Autodesk Inventor part; units mm, degrees
ref_plane "YZ Plane" through (0, 0, 0) normal (1, 0, 0) x (0, 1, 0)
ref_plane "XZ Plane" through (0, 0, 0) normal (0, 1, 0) x (-1, 0, 0)
ref_plane "XY Plane" through (0, 0, 0) normal (0, 0, 1) x (1, 0, 0)
sketch "Sketch1" plane through (0, 0, 0) normal (0, 0, 1) x (1, 0, 0)
  line L0 (-7.2739, -1.4271) -> (7.2739, -1.4271)
  line L1 (7.2739, -1.4271) -> (7.2739, 1.4271)
  line L2 (7.2739, 1.4271) -> (-7.2739, 1.4271)
  line L3 (-7.2739, 1.4271) -> (-7.2739, -1.4271)
  line L4 (-7.2739, -1.4271) -> (7.2739, 1.4271) construction
  line L5 (7.2739, -1.4271) -> (-7.2739, 1.4271) construction
  line L6 (9.525, 3.6783) -> (-9.525, 3.6783)
  line L7 (-9.525, 3.6783) -> (-9.525, 6.4723)
  line L8 (-9.525, 6.4723) -> (9.525, 6.4723)
  line L9 (9.525, 6.4723) -> (9.525, 3.6783)
  line L10 (9.525, 3.6783) -> (-9.525, 6.4723) construction
  line L11 (-9.525, 3.6783) -> (9.525, 6.4723) construction
  line L12 (-7.2739, 1.4271) -> (-9.525, 3.6783)
  line L13 (7.2739, 1.4271) -> (9.525, 3.6783)
  line L14 (-10.922, 5.0753) -> (-8.1026, 7.8947)
  line L15 (-10.922, 5.0753) -> (-6.9348, 5.0753) construction
  line L16 (-10.922, 5.0753) -> (-9.525, 3.6783)
  line L17 (10.922, 5.0753) -> (8.1026, 7.8947)
  line L18 (9.525, 3.6783) -> (10.922, 5.0753)
  line L19 (-8.1026, 7.8947) -> (8.1026, 7.8947)
  line L20 (-19.05, -1.4271) -> (19.05, -1.4271)
  line L21 (19.05, -1.4271) -> (19.05, 15.8839)
  line L22 (19.05, 15.8839) -> (-19.05, 15.8839)
  line L23 (-19.05, 15.8839) -> (-19.05, -1.4271)
  point P0 (0, 0)
  point P1 (0, 5.0753)
  point P2 (0, -1.4271)
  dimension "d0" = 135
  dimension "d1" = 135
  dimension "d2" = 19.05
  dimension "d3" = 2.794
  dimension "d4" = 45
  dimension "d5" = 4.2164
  dimension "d6" = 90
  dimension "d7" = 90
  dimension "d8" = 9.3218
  dimension "d9" = 38.1
extrude "Extrusion1" add sketch "Sketch1" against normal blind 177.8 contours L20 L23 L22 L21 L1 L13 L18 L17 L19 L14 L16 L12 L3
sketch "Sketch2" plane through (0, 0, -177.8) normal (0, 0, -1) x (-1, 0, 0)
  arc A0 (19.05, 29.7163) -> (-19.05, 29.7163) centre (0, 29.7163) ccw
  line L0 (19.05, -1.4271) -> (19.05, 15.8839)
  line L1 (19.05, 15.8839) -> (19.05, -1.4271)
  line L2 (19.05, 15.8839) -> (19.05, 29.7163)
  line L3 (-19.05, -1.4271) -> (-19.05, 15.8839)
  line L4 (-19.05, 15.8839) -> (-19.05, 29.7163)
  line L5 (19.05, 15.8839) -> (-19.05, 15.8839)
  point P0 (0, 0)
extrude "Extrusion2" add sketch "Sketch2" against normal blind 50.8
sketch "Sketch3" plane through (0, 0, -177.8) normal (0, 0, -1) x (-1, 0, 0)
  arc A0 (19.05, 29.7163) -> (-19.05, 29.7163) centre (0, 29.7163) ccw
  point P0 (0, 0)
hole "Hole1" at (0, 29.7163, -177.8) direction (0, 0, 1) diameter 21.6 end through all
fillet "Fillet1" radius 3.175 2 edges at (-19.05, 15.8839, -63.5) (19.05, 15.8839, -63.5)
properties part number "Laser mount 7 inches"
Design review of the part built by this model. Coordinates are the model's own, in mm. A direction names the side the tool comes from. Round coordinates to 2 decimals unless told otherwise and drop trailing zeros. Write each loop counter-clockwise with the first axis right and the second up, starting at its lowest first coordinate (ties: lowest second). Pieces come first, ordered by that corner, then holes.
Item 1: For faces 1 (the flat face through (0, 15.884, -63)), 2 (the cylindrical face through (-0.475, 18.927, -152.044)), 3 (the cylindrical face through (18.095, 14.979, -64.389)), 4 (the flat face through (-7.274, 0, -88)), 5 (the cylindrical face through (-18.145, 14.929, -64.389)), list the 3-axis set-ups (+Z, -Z, +X, -X, +Y, -Y) from which the entire face can be reached by the end or side of a thin tool; tool diameter is ignored.
Item 2: Wall thickness on L1, parallel to Y at x = 0, z = -153; L2, parallel to Y at x = 11, z = -78; L3, parallel to Y at x = -5, z = -113: over which ranges is each line inside the solid? List them lowest first.
Item 3: Consider section A-A on x = 0. Give the boundary of the cut face in (y, z).
Item 4: Consider section C-C on y = 36.5. Give the boundary of the cut face in (x, z).
Item 5: Consider section B-B on z = -61.5. Give the boundary of the cut face in (x, y) (3 decimals).
Item 6: For pin 1 Ø9.5 at (x, z) = (-4, -52) entering from +Y; pin 2 Ø11 at (x, y) = (9, 36.5) entering from +Z, all flat-tipped, find the tip position at first contact; note any pin that passes through.
Item 7: Draft analysis for pull direction X (two halves, no side actions). For faces 6 (the flat face through (9, 39, -127)), 7 (the cylindrical face through (-0.42, 48.76, -152.76)), 8 (the flat face through (7.274, 0, -88)), state which applies: released by +X, released by -X, zero draft, split by the parting line, or undercut.
Check values:
1. face 1: +Z, +X, -X, +Y
1. face 2: +Z, -Z
1. face 3: +Z, +X, +Y
1. face 4: +Z, -Z, -Y
1. face 5: +Z, -X, +Y
2. L1: y = 7.89 to 18.92, 40.52 to 48.77
2. L2: y = -1.43 to 15.88
2. L3: y = 7.89 to 15.88
3. outline: (7.89, -177.8) - (18.92, -177.8) - (18.92, -127) - (15.88, -127) - (15.88, 0) - (7.89, 0) - close; (40.52, -177.8) - (48.77, -177.8) - (48.77, -127) - (40.52, -127) - close
4. outline: (-17.8, -177.8) - (-8.4, -177.8) - (-8.4, -127) - (-17.8, -127) - close; (8.4, -177.8) - (17.8, -177.8) - (17.8, -127) - (8.4, -127) - close
5. outline: (-19.05, -1.427) - (-7.274, -1.427) - (-7.274, 1.427) - (-9.525, 3.678) - (-10.922, 5.075) - (-8.103, 7.895) - (8.103, 7.895) - (10.922, 5.075) - (9.525, 3.678) - (7.274, 1.427) - (7.274, -1.427) - (19.05, -1.427) - (19.05, 12.709) arc R3.175 ccw to (15.875, 15.884) - (-15.875, 15.884) arc R3.175 ccw to (-19.05, 12.709) - close
6. pin 1: stops at y = 15.88
6. pin 2: stops at z = -127
7. face 6: zero draft
7. face 7: split by the parting line
7. face 8: undercut
